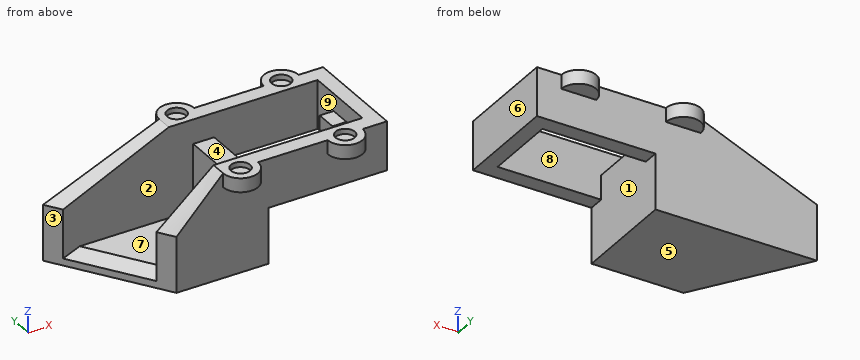
Autodesk Fusion 360 part; units mm, degrees
sketch "Base" plane through (0, 0, 0) normal (0, 0, 1) x (1, 0, 0)
  line L0 (0, 0) -> (46.334, 0)
  line L1 (46.334, 0) -> (46.334, 30)
  line L2 (46.334, 30) -> (0, 30)
  line L3 (0, 30) -> (0, 0)
  dimension "d2" = 46.334
  dimension "d3" = 30
extrude "Extrude1" add sketch "Base" along normal blind 4
sketch "Side Profile" plane through (0, 0, 0) normal (0, -1, 0) x (1, 0, 0)
  line L0 (0, 0) -> (46.334, 0)
  line L1 (46.334, 0) -> (46.334, 4)
  line L2 (46.334, 4) -> (0, 4)
  line L3 (0, 4) -> (0, 0)
  line L4 (46.334, 4) -> (46.334, 16)
  line L5 (46.334, 16) -> (80.334, 16)
  line L6 (80.334, 16) -> (80.334, 30)
  line L7 (80.334, 30) -> (0, 30)
  line L8 (0, 30) -> (0, 4)
  dimension "d6" = 12
  dimension "d7" = 34
  dimension "d8" = 14
  dimension "d11" = 46.334
  dimension "d52" = 80.334
extrude "Extrude2" add sketch "Side Profile" against normal blind 4.5 contours L2 L4 L5 L6 L7 L8
extrude "Extrude3" add sketch "Side Profile" against normal blind 4.5 from surface at -25.5 contours L2 L4 L5 L6 L7 L8
sketch "Front End" plane through (0, 0, 0) normal (0, -1, 0) x (1, 0, 0)
  line L0 (0, 0) -> (46.334, 0)
  line L1 (46.334, 0) -> (46.334, 16)
  line L2 (46.334, 16) -> (80.334, 16)
  line L3 (80.334, 16) -> (80.334, 30)
  line L4 (80.334, 30) -> (0, 30)
  line L5 (0, 30) -> (0, 0)
  line L6 (80.334, 30) -> (76.034, 30)
  line L7 (76.034, 30) -> (76.034, 16)
  line L8 (76.034, 16) -> (80.334, 16)
  line L9 (80.334, 16) -> (80.334, 30)
  dimension "d17" = 4.3
extrude "Extrude4" add sketch "Front End" against normal blind 30 contours L2 L3 L4 L6 L7 L8 L9
sketch "Middle End" plane through (0, 0, 0) normal (0, -1, 0) x (1, 0, 0)
  line L0 (80.334, 30) -> (0, 30)
  line L1 (0, 30) -> (0, 0)
  line L2 (0, 0) -> (46.334, 0)
  line L3 (46.334, 0) -> (46.334, 16)
  line L4 (46.334, 16) -> (80.334, 16)
  line L5 (80.334, 16) -> (80.334, 30)
  line L6 (46.334, 23) -> (40.334, 23)
  line L7 (40.334, 23) -> (40.334, 0)
  line L8 (40.334, 0) -> (46.334, 0)
  line L9 (46.334, 0) -> (46.334, 23)
  dimension "d20" = 7
  dimension "d21" = 6
extrude "Extrude5" add sketch "Middle End" against normal blind 30 contours L2 L3 L6 L7 L8 L9
sketch "Lip" plane through (76.034, 0, 0) normal (-1, 0, 0) x (0, -1, 0)
  line L0 (-25.5, 30) -> (-25.5, 16)
  line L1 (-25.5, 16) -> (-4.5, 16)
  line L2 (-4.5, 16) -> (-4.5, 30)
  line L3 (-4.5, 30) -> (-25.5, 30)
  line L4 (-18, 25) -> (-12, 25)
  line L5 (-12, 25) -> (-12, 21)
  line L6 (-12, 21) -> (-18, 21)
  line L7 (-18, 21) -> (-18, 25)
  dimension "d24" = 5
  dimension "d25" = 6
  dimension "d26" = 4
  dimension "d27" = 7.5
extrude "Extrude6" add sketch "Lip" along normal blind 4 contours L4 L5 L6 L7
sketch "Magnet Holders" plane through (0, 0, 30) normal (0, 0, 1) x (-1, 0, 0)
  line L0 (-80.334, -30) -> (0, -30)
  line L1 (0, -30) -> (0, -25.5)
  line L2 (0, -25.5) -> (-76.034, -25.5)
  line L3 (-76.034, -25.5) -> (-76.034, -4.5)
  line L4 (-76.034, -4.5) -> (0, -4.5)
  line L5 (0, -4.5) -> (0, 0)
  line L6 (0, 0) -> (-80.334, 0)
  line L7 (-80.334, 0) -> (-80.334, -30)
  circle A0 centre (-68.334, -30) radius 5
  circle A1 centre (-38.334, -30) radius 5
  circle A2 centre (-38.334, 0) radius 5
  circle A3 centre (-68.334, 0) radius 5
  circle A4 centre (-38.334, 0) radius 2.75
  circle A5 centre (-68.334, 0) radius 2.75
  circle A6 centre (-38.334, -30) radius 2.75
  circle A7 centre (-68.334, -30) radius 2.75
  dimension "d33" = 10
  dimension "d34" = 10
  dimension "d35" = 10
  dimension "d36" = 10
  dimension "d37" = 12
  dimension "d38" = 12
  dimension "d43" = 5.5
  dimension "d44" = 5.5
  dimension "d45" = 5.5
  dimension "d46" = 5.5
  dimension "d50" = 42
  dimension "d51" = 42
extrude "Extrude8" add sketch "Magnet Holders" against normal blind 4 contours L0 A7 | L0 A0 A7 | L0 A1 A6 | L0 A6 | L6 A3 A5 | L6 A5 | L6 A2 A4 | L6 A4 picked at (-68.2655, -30.9141) picked at (-37.4674, -30.6679) picked at (-68.2655, 0.9141) picked at (-39.0365, 1.0303)
extrude "Extrude9" cut sketch "Magnet Holders" against normal blind 1.5 contours L0 A7 | L0 A7 | L0 A6 | L0 A6 | L6 A5 | L6 A5 | L6 A4 | L6 A4
sketch "Conduit Angle" plane through (0, 0, 30) normal (0, 0, 1) x (-1, 0, 0)
  circle A0 centre (-68.334, 0) radius 2.75
  circle A1 centre (-38.334, -30) radius 2.75
  circle A2 centre (-38.334, 0) radius 2.75
  circle A3 centre (-68.334, -30) radius 2.75
  line L0 (-33.334, -30) -> (0, -30)
  line L1 (0, -30) -> (0, -25.5)
  line L2 (0, -25.5) -> (-76.034, -25.5)
  line L3 (-76.034, -25.5) -> (-76.034, -4.5)
  line L4 (-76.034, -4.5) -> (0, -4.5)
  line L5 (0, -4.5) -> (0, 0)
  line L6 (0, 0) -> (-33.334, 0)
  arc A4 (-33.334, 0) -> (-43.334, 0) centre (-38.334, 0) ccw
  line L7 (-43.334, 0) -> (-63.334, 0)
  arc A5 (-63.334, 0) -> (-73.334, 0) centre (-68.334, 0) ccw
  line L8 (-73.334, 0) -> (-80.334, 0)
  line L9 (-80.334, 0) -> (-80.334, -30)
  line L10 (-80.334, -30) -> (-73.334, -30)
  arc A6 (-73.334, -30) -> (-63.334, -30) centre (-68.334, -30) ccw
  line L11 (-63.334, -30) -> (-43.334, -30)
  arc A7 (-43.334, -30) -> (-33.334, -30) centre (-38.334, -30) ccw
  line L12 (-40.334, -4.5) -> (-40.334, -25.5)
  line L13 (-40.334, -25.5) -> (0, -25.5)
  line L14 (0, -25.5) -> (0, -4.5)
  line L15 (0, -4.5) -> (-40.334, -4.5)
  line L16 (0, -30) -> (-19.932, 0)
  dimension "d53" = 33.6
extrude "Extrude10" cut sketch "Conduit Angle" against normal blind 30 contours L1 L2 L13 L16 | L2 L4 L13 L14 L15 L16 | L4 L5 L6 L15 L16
sketch "Conduit Height" plane through (13.8279, 9.1873, 0) normal (-0.8329, -0.5534, 0) x (0.5534, -0.8329, 0)
  line L0 (-19.585, 4) -> (-19.585, 30)
  line L1 (-19.585, 30) -> (-24.9876, 30)
  line L2 (-24.9876, 30) -> (-24.9876, 0)
  line L3 (-24.9876, 0) -> (11.0302, 0)
  line L4 (11.0302, 0) -> (11.0302, 30)
  line L5 (11.0302, 30) -> (5.6275, 30)
  line L6 (5.6275, 30) -> (5.6275, 4)
  line L7 (5.6275, 4) -> (-19.585, 4)
  line L8 (-24.9876, 0) -> (11.0302, 0)
  line L9 (11.0302, 0) -> (11.0302, 16)
  line L10 (11.0302, 16) -> (-24.9876, 16)
  line L11 (-24.9876, 16) -> (-24.9876, 0)
  point P0 (5.6275, 16)
  point P1 (-19.585, 16)
  dimension "d56" = 16
sketch "Colour Sensor Cover Shape" plane through (0, 0, 30) normal (0, 0, 1) x (-1, 0, 0)
  line L0 (0, -30) -> (-2.9898, -25.5)
  line L1 (-2.9898, -25.5) -> (-76.034, -25.5)
  line L2 (-76.034, -25.5) -> (-76.034, -4.5)
  line L3 (-76.034, -4.5) -> (-16.9422, -4.5)
  line L4 (-16.9422, -4.5) -> (-19.932, 0)
  line L5 (-19.932, 0) -> (-33.334, 0)
  arc A0 (-33.334, 0) -> (-43.334, 0) centre (-38.334, 0) ccw
  line L6 (-43.334, 0) -> (-63.334, 0)
  arc A1 (-63.334, 0) -> (-73.334, 0) centre (-68.334, 0) ccw
  line L7 (-73.334, 0) -> (-80.334, 0)
  line L8 (-80.334, 0) -> (-80.334, -30)
  line L9 (-80.334, -30) -> (-73.334, -30)
  arc A2 (-73.334, -30) -> (-63.334, -30) centre (-68.334, -30) ccw
  line L10 (-63.334, -30) -> (-43.334, -30)
  arc A3 (-43.334, -30) -> (-33.334, -30) centre (-38.334, -30) ccw
  line L11 (-33.334, -30) -> (0, -30)
  circle A4 centre (-68.334, 0) radius 2.75
  circle A5 centre (-38.334, -30) radius 2.75
  circle A6 centre (-38.334, 0) radius 2.75
  circle A7 centre (-68.334, -30) radius 2.75
  line L12 (-33.334, -30) -> (-33.334, 0)
  point P0 (-33.334, -25.5)
  point P1 (-33.334, -4.5)
sketch "Right Loft Outside Shape" plane through (0, 0, 0) normal (0, -1, 0) x (1, 0, 0)
  line L0 (19.932, 30) -> (19.932, 0)
  line L1 (19.932, 0) -> (46.334, 0)
  line L2 (46.334, 0) -> (46.334, 16)
  line L3 (46.334, 16) -> (80.334, 16)
  line L4 (80.334, 16) -> (80.334, 30)
  line L5 (80.334, 30) -> (73.334, 30)
  line L6 (73.334, 30) -> (73.334, 26)
  line L7 (73.334, 26) -> (63.334, 26)
  line L8 (63.334, 26) -> (63.334, 30)
  line L9 (63.334, 30) -> (43.334, 30)
  line L10 (43.334, 30) -> (43.334, 26)
  line L11 (43.334, 26) -> (33.334, 26)
  line L12 (33.334, 26) -> (33.334, 30)
  line L13 (33.334, 30) -> (19.932, 30)
  line L14 (33.334, 30) -> (19.932, 16)
  point P0 (33.334, 30)
  point P1 (19.932, 16)
sketch "Right Loft Inside Shape" plane through (0, 4.5, 0) normal (0, 1, 0) x (-1, 0, 0)
  line L0 (-16.9422, 4) -> (-16.9422, 30)
  line L1 (-16.9422, 30) -> (-76.034, 30)
  line L2 (-76.034, 30) -> (-76.034, 16)
  line L3 (-76.034, 16) -> (-46.334, 16)
  line L4 (-46.334, 16) -> (-46.334, 23)
  line L5 (-46.334, 23) -> (-40.334, 23)
  line L6 (-40.334, 23) -> (-40.334, 4)
  line L7 (-40.334, 4) -> (-16.9422, 4)
  line L8 (-33.334, 30) -> (-16.9422, 16)
  point P0 (-33.334, 30)
  point P1 (-16.9422, 16)
sketch "Left Loft Inside Shape" plane through (0, 25.5, 0) normal (0, -1, 0) x (1, 0, 0)
  line L0 (2.9898, 30) -> (2.9898, 4)
  line L1 (2.9898, 4) -> (40.334, 4)
  line L2 (40.334, 4) -> (40.334, 23)
  line L3 (40.334, 23) -> (46.334, 23)
  line L4 (46.334, 23) -> (46.334, 16)
  line L5 (46.334, 16) -> (76.034, 16)
  line L6 (76.034, 16) -> (76.034, 30)
  line L7 (76.034, 30) -> (2.9898, 30)
  line L8 (33.334, 30) -> (2.9898, 16)
  point P0 (33.334, 30)
  point P1 (2.9898, 16)
sketch "Left Loft Outside Shape" plane through (0, 30, 0) normal (0, 1, 0) x (-1, 0, 0)
  line L0 (-33.334, 30) -> (-33.334, 26)
  line L1 (-33.334, 26) -> (-43.334, 26)
  line L2 (-43.334, 26) -> (-43.334, 30)
  line L3 (-43.334, 30) -> (-63.334, 30)
  line L4 (-63.334, 30) -> (-63.334, 26)
  line L5 (-63.334, 26) -> (-73.334, 26)
  line L6 (-73.334, 26) -> (-73.334, 30)
  line L7 (-73.334, 30) -> (-80.334, 30)
  line L8 (-80.334, 30) -> (-80.334, 16)
  line L9 (-80.334, 16) -> (-46.334, 16)
  line L10 (-46.334, 16) -> (-46.334, 0)
  line L11 (-46.334, 0) -> (0, 0)
  line L12 (0, 0) -> (0, 30)
  line L13 (0, 30) -> (-33.334, 30)
  line L14 (-33.334, 30) -> (0, 16)
  point P0 (-33.334, 30)
  point P1 (0, 16)
loft "Loft1" cut profiles "Right Loft Outside Shape", "Right Loft Inside Shape" section 1 contours L0 L13 L14 section 2 contours L0 L1 L8
loft "Loft2" cut profiles "Left Loft Inside Shape", "Left Loft Outside Shape" section 1 contours L0 L7 L8 section 2 contours L12 L13 L14
chamfer "Chamfer2" distance 4 distance2 2 1 edges at (9.966, 15, 4) measured on face at (20.0887, 18.5, 4)
equation "base_plate_thickness = 4 mm"
equation "d4 = base_plate_thickness"
equation "d37 = 7 mm + 5 mm"
equation "d38 = 7 mm + 5 mm"
Check sheet for the modelled part. Datum: model origin and axes. Units: mm. Face numbers are marked on the shaded views. A direction names the side the tool comes from. Round coordinates to 2 decimals unless told otherwise and drop trailing zeros. Order: outer loops, then holes, each group sorted by start corner. A loop starts at its lowest first (then second) coordinate and runs counter-clockwise, first axis right, second up. Notation, with made-up numbers: M 31,30 L 62,30 A24 cw 62,48 Z; hole C 53.25,-8 d1. An arc over 180 degrees is marked long. Answer in a Markdown table with one row per item.
(1) Section check C-C on z = 14. Record the boundary of the cut face in (x, y).
Findings:
| item | result |
|---|---|
| outline | M 0,30 L 2.99,25.5 L 40.33,25.5 L 40.33,4.5 L 16.94,4.5 L 19.93,0 L 46.33,0 L 46.33,30 Z |
(2) Section check D-D on y = 22. Record the boundary of the cut face in (x, z).
Findings:
| item | result |
|---|---|
| outline | M 5.32,0 L 46.33,0 L 46.33,23 L 40.33,23 L 40.33,4 L 10.12,4 L 5.32,2 Z; M 76.03,16 L 80.33,16 L 80.33,30 L 76.03,30 Z |
(3) Section check B-B on y = 14. Record the boundary of the cut face in (x, z).
Findings:
| item | result |
|---|---|
| outline | M 10.63,0 L 46.33,0 L 46.33,23 L 40.33,23 L 40.33,4 L 15.43,4 L 10.63,2 Z; M 72.03,21 L 76.03,21 L 76.03,16 L 80.33,16 L 80.33,30 L 76.03,30 L 76.03,25 L 72.03,25 Z |
(4) Draft check along X on the marked faces 6, 7, 8 and 9. Enter one of: +X half, -X half, draft (parallel to the pull), parting line (faces both ways), or undercut.
Findings:
| item | result |
|---|---|
| face 6 | +X half |
| face 7 | draft |
| face 8 | undercut |
| face 9 | undercut |
(5) Material ranges on line 1 along Y through (x, z) = (51, 25); line 2 along X through (y, z) = (19.5, 26); line 3 along Z through (x, y) = (37, 22), recorded low to high. Write a range as from..to.
Findings:
| item | result |
|---|---|
| line 1 | y = 0..4.5, 25.5..30 |
| line 2 | x = 76.03..80.33 |
| line 3 | z = 0..4 |
(6) Gauge pin test, flat ends, axial feed: pin 1 (1 mm diameter, centred on x = 34, y = 9, fed in from +Z); pin 2 (3 mm diameter, centred on x = 37.5, y = 0, fed in from +Z); pin 3 (11 mm diameter, centred on y = 13.5, z = 25.5, fed in from -X). Record the tip position at first contact, or that the pin passes through.
Findings:
| item | result |
|---|---|
| pin 1 | stops at z = 4 |
| pin 2 | stops at z = 28.5 |
| pin 3 | stops at x = 40.33 |
(7) Set-up check for the marked faces 1, 2, 3, 4 and 5: record each of +Z, -Z, +X, -X, +Y, -Y from which the full face is reachable in a straight line by a thin tool's end or side.
Findings:
| item | result |
|---|---|
| face 1 | -Z |
| face 2 | +Z |
| face 3 | +Z, -Z, -X, -Y |
| face 4 | +Z, -X |
| face 5 | -Z, +X, -X, +Y, -Y |
(8) Section check A-A on x = 62. Record the boundary of the cut face in (y, z), plus the area to 3 significant figures.
Findings:
| item | result |
|---|---|
| outline | M 0,16 L 4.5,16 L 4.5,30 L 0,30 Z; M 25.5,16 L 30,16 L 30,30 L 25.5,30 Z |
| area | 126 mm^2 |
